```python
from build123d import *

# Parameters (mm, degrees)
EXTRUDE_2_DEPTH      = 4
SKETCH_2_R           = 1.5
CUT_EXTRUDE_1_DEPTH  = 10
SKETCH_4_W           = 100
SKETCH_4_H           = 10
CUT_EXTRUDE_2_DEPTH  = 10
FILLET_1_R           = 5
SKETCH_5_R           = 1.5
CUT_EXTRUDE_3_DEPTH  = 6
SKETCH_7_W           = 4
SKETCH_7_H           = 25.94
EXTRUDE_3_DEPTH      = 2
FILLET_5_R           = 1
SKETCH_9_R           = 1.5
CUT_EXTRUDE_6_DEPTH  = 10
SKETCH_13_R          = 1.5
CUT_EXTRUDE_8_DEPTH  = 10
CUT_EXTRUDE_9_DEPTH  = 4
FILLET_9_R           = 2
SKETCH_15_W          = 4
SKETCH_15_H          = 25.94
CUT_EXTRUDE_12_DEPTH = 10
SKETCH_16_W          = 77
SKETCH_16_H          = 26
CUT_EXTRUDE_13_DEPTH = 10
FILLET_10_R          = 5


with BuildPart() as part:
    # 草图1 → 凸台-拉伸2 (new body)
    with BuildSketch(Plane.XY):
        Polygon((0, 0), (0, 36), (35, 36), (135, 36), (135, 16.447466896), (135, 0), align=None)
    extrude(amount=EXTRUDE_2_DEPTH)

    # 草图2 → 切除-拉伸1 (cut)
    with BuildSketch(Plane.XY.offset(4)):
        with Locations((3, 4)):
            Circle(SKETCH_2_R)
        with Locations((3, 24)):
            Circle(SKETCH_2_R)
    extrude(amount=-CUT_EXTRUDE_1_DEPTH, mode=Mode.SUBTRACT)

    # 草图4 → 切除-拉伸2 (cut)
    with BuildSketch(Plane.XY.offset(4)):
        with Locations((85, 5)):
            Rectangle(SKETCH_4_W, SKETCH_4_H)
    extrude(amount=-CUT_EXTRUDE_2_DEPTH, mode=Mode.SUBTRACT)

    # 圆角1
    fillet_1_edges = [part.edges().sort_by_distance(p)[0] for p in [
        (35, 10, 2),
        (135, 10, 2),
        (135, 36, 2),
        (0, 36, 2),
        (0, 0, 2),
        (35, 0, 2),
    ]]
    fillet(fillet_1_edges, radius=FILLET_1_R - 0.0001)  # a hair under: the kernel refuses the full size

    # 草图5 → 切除-拉伸3 (cut)
    with BuildSketch(Plane.XY.offset(4)):
        with Locations((97.5, 33)):
            Circle(SKETCH_5_R)
        with Locations((53, 33)):
            Circle(SKETCH_5_R)
        with Locations((77.5, 33)):
            Circle(SKETCH_5_R)
    extrude(amount=-CUT_EXTRUDE_3_DEPTH, mode=Mode.SUBTRACT)

    # 草图7 → 凸台-拉伸3 (add)
    with BuildSketch(Plane.XY.offset(4)):
        with Locations((-2, 18)):
            Rectangle(SKETCH_7_W, SKETCH_7_H)
    extrude(amount=-EXTRUDE_3_DEPTH)

    # 圆角5
    fillet_5_edges = [part.edges().sort_by_distance(p)[0] for p in [
        (-4, 5.03, 3),
        (-4, 30.97, 3),
    ]]
    fillet(fillet_5_edges, radius=FILLET_5_R)

    # 草图9 → 切除-拉伸6 (cut)
    with BuildSketch(Plane.XY.offset(4)):
        with Locations((110, 17)):
            Circle(SKETCH_9_R)
    extrude(amount=-CUT_EXTRUDE_6_DEPTH, mode=Mode.SUBTRACT)

    # 草图13 → 切除-拉伸8 (cut)
    with BuildSketch(Plane.XY.offset(4)):
        with Locations((33, 33)):
            Circle(SKETCH_13_R)
    extrude(amount=-CUT_EXTRUDE_8_DEPTH, mode=Mode.SUBTRACT)

    # 草图11 → 切除-拉伸9 (cut)
    with BuildSketch(Plane.XY.offset(4)):
        Polygon((31, 4), (14, 32), (31, 32), align=None)
        Polygon((8, 4), (24, 4), (8, 29), align=None)
    extrude(amount=-CUT_EXTRUDE_9_DEPTH, mode=Mode.SUBTRACT)

    # 圆角9
    fillet_9_edges = [part.edges().sort_by_distance(p)[0] for p in [
        (8, 29, 2),
        (8, 4, 2),
        (24, 4, 2),
        (31, 4, 2),
        (14, 32, 2),
        (31, 32, 2),
    ]]
    fillet(fillet_9_edges, radius=FILLET_9_R)

    # 草图15 → 切除-拉伸12 (cut)
    with BuildSketch(Plane.XY.offset(4)):
        with Locations((-2, 18)):
            Rectangle(SKETCH_15_W, SKETCH_15_H)
    extrude(amount=-CUT_EXTRUDE_12_DEPTH, mode=Mode.SUBTRACT)

    # 草图16 → 切除-拉伸13 (cut)
    with BuildSketch(Plane.XY.offset(4)):
        with Locations((96.5, 23)):
            Rectangle(SKETCH_16_W, SKETCH_16_H)
    extrude(amount=-CUT_EXTRUDE_13_DEPTH, mode=Mode.SUBTRACT)

    # 圆角10
    fillet_10_edges = [part.edges().sort_by_distance(p)[0] for p in [
        (58, 36, 2),
        (58, 10, 2),
    ]]
    fillet(fillet_10_edges, radius=FILLET_10_R)


solid = part.part
```
Build history of the part. All positions in model axes, mm. A direction names the side the tool comes from. Coordinates: 2 decimals unless noted, no trailing zeros. Order: outer loops, then holes, each group sorted by start corner. A loop starts at its lowest first (then second) coordinate and runs counter-clockwise, first axis right, second up. Notation, with made-up numbers: M 43,-8.75 L 68,-8.75 A18 ccw 68,13.25 Z; hole C -39.75,-28.5 d10. An arc over 180 degrees is marked long. One line per question, with ' | ' between items. Start each with the question number.
1. Cut at B-B (z = 0.95). Count the separate pieces of the cut face and the enclosed holes in it, plus the area to 3 significant figures.
2. Cut at A-A (x = 33). Write the cut outline in (y, z).
3. Cut at D-D (x = 3). Write the cut outline in (y, z).
4. Wall check: line 1 along Y through (x, z) = (53, 1.35); line 2 along Y through (x, z) = (2, 1.95); line 3 along X through (y, z) = (21.5, 3.7) (3 decimals). Give the ranges that are in metal, low to high. Write a range as [from, to].
5. Mould opens along Y. For faces 4 (the face through (0, 18, 2)), 5 (the face through (29.5, 9.21, 1.97)), 6 (the face through (1, 2, 2)) say: +Y half, -Y half, draft (parallel to the pull), parting line (faces both ways), or undercut.
6. Flat gauge pin, fed straight in: P1, Ø2.5, axis at x = 53, y = 33, coming from the -Z side. Where does the tip first touch, or does it go through?
7. Cut at C-C (y = 19.5). Write the cut outline in (x, z), plus the area to 3 significant figures.
8. Tool access for faces 1 (the face through (46, 10, 2)), 2 (the face through (36, 22, 4)), 3 (the face through (31, 21, 2)): list every direction of +Z, -Z, +X, -X, +Y, -Y with a clear straight run to the whole face (end or side of a thin tool).
The answers:
1) separate pieces: 1 | enclosed holes: 6 | area: 1,400 mm2
2) outline: M 1,0 L 31.5,0 L 31.5,4 L 1,4 Z; M 34.5,0 L 36,0 L 36,4 L 34.5,4 Z
3) outline: M 0.42,0 L 2.5,0 L 2.5,4 L 0.42,4 Z; M 5.5,0 L 22.5,0 L 22.5,4 L 5.5,4 Z; M 25.5,0 L 35.58,0 L 35.58,4 L 25.5,4 Z
4) line 1: y = [10, 31.5], [34.5, 36] | line 2: y = [1, 2.88], [5.12, 22.88], [25.12, 35] | line 3: x = [0, 8], [12.8, 20.375], [31, 58]
5) face 4: draft | face 5: undercut | face 6: -Y half
6) P1: passes through
7) outline: M 0,0 L 8,0 L 8,4 L 0,4 Z; M 14.08,0 L 21.59,0 L 21.59,4 L 14.08,4 Z; M 31,0 L 58,0 L 58,4 L 31,4 Z | area: 170 mm2
8) face 1: +Z, -Z, +X, -Y | face 2: +Z, +X, -X, +Y, -Y | face 3: +Z, -Z
